```python
from build123d import *

# Parameters (mm, degrees)
F3_DEPTH      = 61.9125
F5_DEPTH      = 50.8
F5_DEPTH_BACK = 3.175


with BuildPart() as f3:
    # F2 (on offset) → F3 (new body)
    with BuildSketch(Plane.XZ.offset(-3.175)):
        Polygon((0, 2054.225), (0, 0), (19.05, 0), (31.75, 0), (31.75, 2041.525), (926.30625, 2041.525), (926.30625, 0), (939.00625, 0), (958.05625, 0), (958.05625, 2054.225), (958.05625, 2073.275), (0, 2073.275), align=None)
    extrude(amount=-F3_DEPTH)

    # F4 (on Front) → F5 (join, two sides)
    with BuildSketch(Plane.XZ) as f5_sk:
        Polygon((0, 2054.225), (0, 0), (19.05, 0), (19.05, 2041.525), (19.05, 2054.225), (364.33125, 2054.225), (593.725, 2054.225), (939.00625, 2054.225), (939.00625, 2041.525), (939.00625, 0), (958.05625, 0), (958.05625, 2054.225), (958.05625, 2073.275), (0, 2073.275), align=None)
    extrude(amount=F5_DEPTH)
    extrude(f5_sk.sketch, amount=-F5_DEPTH_BACK)


solid = f3.part
```
Verification items for the finished model (mm, model axes). A direction names the side the tool comes from. Round coordinates to 2 decimals unless told otherwise and drop trailing zeros. Write each loop counter-clockwise with the first axis right and the second up, starting at its lowest first coordinate (ties: lowest second). Pieces come first, ordered by that corner, then holes. Notation, with made-up numbers: (-22, 79.5) -> (4, 79.5) arc R11 cw to (4, 100.5) -> close; hole circle Ø4 at (58, 8.25). An arc over 180 degrees is marked (long way). Write each question's results on one line, items separated by ' | '. Start each with the question number.
1. Set-up check for faces 5 (the flat face through (16, -50.8, 1041)), 6 (the flat face through (19.05, -24, 1013)), 7 (the flat face through (473, 34, 2041.525)): record each of +Z, -Z, +X, -X, +Y, -Y from which the full face is reachable in a straight line by a thin tool's end or side.
2. Cross-section at C-C (x = 655). Enter the section's corners in (y, z) (1 decimal).
3. Draft check along X on faces 1 (the flat face through (0, 6, 1051)), 2 (the flat face through (958.056, 6, 1022)), 3 (the flat face through (473, -24, 2054.225)), 4 (the flat face through (16, 65.088, 1041)). Enter one of: +X half, -X half, draft (parallel to the pull), parting line (faces both ways), or undercut.
4. Cross-section at B-B (y = 27). Enter the section's corners in (x, z) (3 decimals), then the cut area to 3 significant figures.
5. Material ranges on probe 1 along X at (y, z) = (56.5, 1639); probe 2 along X at (y, z) = (-36, 1746); probe 3 along Z at (x, y) = (472, -39) (3 decimals), recorded low to high. Write a range as from..to.
Solutions:
1) face 5: +Z, -Z, +X, -X, -Y | face 6: -Z, -Y | face 7: -Z, +Y, -Y
2) outline: (-50.8, 2054.2) -> (3.2, 2054.2) -> (3.2, 2041.5) -> (65.1, 2041.5) -> (65.1, 2073.3) -> (-50.8, 2073.3) -> close
3) face 1: -X half | face 2: +X half | face 3: undercut | face 4: draft
4) outline: (0, 0) -> (31.75, 0) -> (31.75, 2041.525) -> (926.306, 2041.525) -> (926.306, 0) -> (958.056, 0) -> (958.056, 2073.275) -> (0, 2073.275) -> close | area: 160,000 mm2
5) probe 1: x = 0..31.75, 926.31..958.06 | probe 2: x = 0..19.05, 939.01..958.06 | probe 3: z = 2054.225..2073.275
